from build123d import *

# Parameters (mm, degrees)
SKETCH1_R               = 50.8
SKETCH1_R_2             = 3.175
BOSS_EXTRUDE1_DEPTH     = 71.12
CUT_EXTRUDE1_DEPTH      = 102.09072361
CUT_EXTRUDE1_DEPTH_BACK = 102.09072361
SKETCH2_R               = 1.27
SKETCH7_R               = 2.5
CUT_EXTRUDE4_DEPTH      = 12.7
SKETCH8_R               = 15.748
SKETCH8_R_2             = 3.175
BOSS_EXTRUDE2_DEPTH     = 6.35
CUT_EXTRUDE6_DEPTH      = 4
SKETCH6_R               = 2.5
CUT_EXTRUDE7_DEPTH      = 7


with BuildPart() as part:
    # Sketch1 → Boss-Extrude1 (new body)
    with BuildSketch(Plane.XY):
        Circle(SKETCH1_R)
        Circle(SKETCH1_R_2, mode=Mode.SUBTRACT)
    extrude(amount=BOSS_EXTRUDE1_DEPTH)

    # Sketch2 → Cut-Extrude1 (cut, two sides: drawn at the far end of the back side and taken through both)
    with BuildSketch(Plane(origin=(0, 0, 0), x_dir=(0, 0, -1), z_dir=(1, 0, 0)).offset(-CUT_EXTRUDE1_DEPTH_BACK)):
        with Locations((-35.56, 38.1)):
            Circle(SKETCH2_R)
    extrude(amount=CUT_EXTRUDE1_DEPTH + CUT_EXTRUDE1_DEPTH_BACK, mode=Mode.SUBTRACT)

    # Sketch7 → Cut-Extrude4 (cut)
    with BuildSketch(Plane(origin=(0, 0, 0), x_dir=(-1, 0, 0), z_dir=(0, 0, -1))):
        with Locations((28.575, 0)):
            Circle(SKETCH7_R)
        with Locations((0, 28.575)):
            Circle(SKETCH7_R)
        with Locations((-28.575, 0)):
            Circle(SKETCH7_R)
        with Locations((0, -28.575)):
            Circle(SKETCH7_R)
    cut_extrude4 = extrude(amount=-CUT_EXTRUDE4_DEPTH, mode=Mode.SUBTRACT)

    # Mirror1: Cut-Extrude4 across plane
    add(cut_extrude4.mirror(Plane.XY.offset(35.56)), mode=Mode.SUBTRACT)

    # Sketch8 → Boss-Extrude2 (add)
    with BuildSketch(Plane.XY.offset(71.12)):
        Circle(SKETCH8_R)
        Circle(SKETCH8_R_2, mode=Mode.SUBTRACT)
    extrude(amount=BOSS_EXTRUDE2_DEPTH)

    # Sketch5 → Cut-Extrude6 (cut)
    with BuildSketch(Plane.XY.offset(77.47)):
        with BuildLine():
            Line((-4.330127019, 5.5), (4.330127019, 5.5))
            ThreePointArc((4.330127019, 5.5), (7, 0), (4.330127019, -5.5))
            Line((4.330127019, -5.5), (-4.330127019, -5.5))
            ThreePointArc((-4.330127019, -5.5), (-7, 0), (-4.330127019, 5.5))
        make_face()
    extrude(amount=-CUT_EXTRUDE6_DEPTH, mode=Mode.SUBTRACT)

    # Sketch6 → Cut-Extrude7 (cut)
    with BuildSketch(Plane.XY.offset(77.47)):
        with Locations((-8, 8)):
            Circle(SKETCH6_R)
        with Locations((8, 8)):
            Circle(SKETCH6_R)
        with Locations((8, -8)):
            Circle(SKETCH6_R)
        with Locations((-8, -8)):
            Circle(SKETCH6_R)
    extrude(amount=-CUT_EXTRUDE7_DEPTH, mode=Mode.SUBTRACT)

    # Sketch9 → Cut-Revolve1 (revolve, cut)
    with BuildSketch(Plane(origin=(0, 0, 0), x_dir=(0, 0, -1), z_dir=(1, 0, 0)), mode=Mode.PRIVATE) as cut_revolve1_sk:
        with BuildLine():
            Line((-71.12, 50.8), (-46.204077708, 45.460873794))
            ThreePointArc((-46.204077708, 45.460873794), (-35.56, 44.33323643), (-24.915922292, 45.460873794))
            Line((-24.915922292, 45.460873794), (0, 50.8))
            Line((0, 50.8), (-71.12, 50.8))
        make_face()
    revolve(cut_revolve1_sk.sketch.rotate(Axis((0, 0, -3.8735), (0, 0, 1)), 90), axis=Axis((0, 0, -3.8735), (0, 0, 1)), mode=Mode.SUBTRACT)


solid = part.part
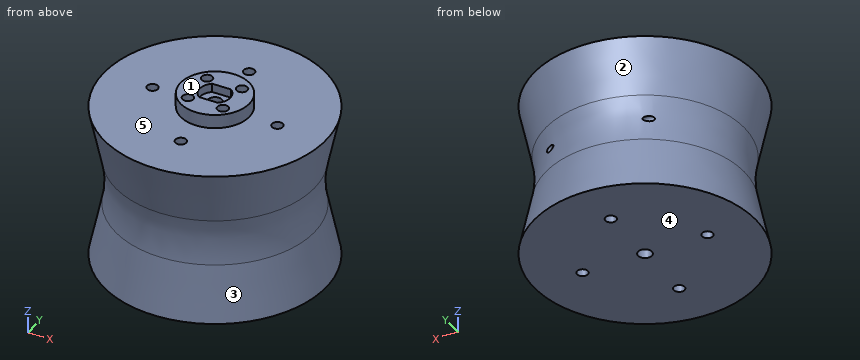
Could you check a few things on this model? Use its own coordinates, in mm. Face numbers are marked on the shaded views. A direction names the side the tool comes from. Round coordinates to 2 decimals unless told otherwise and drop trailing zeros. Write each loop counter-clockwise with the first axis right and the second up, starting at its lowest first coordinate (ties: lowest second). Pieces come first, ordered by that corner, then holes. Notation, with made-up numbers: (59.5, 6) - (117.5, 6) arc R25 ccw to (117.5, 29) - close; hole circle Ø4 at (13.5, 38.25). An arc over 180 degrees is marked (long way). Use a Markdown table: item, result.
Q1. Please list where these lines run through material, in increasing order: L1, parallel to Y at x = -8, z = 74.5; L2, parallel to Y at x = 9, z = 70.5; L3, parallel to Y at x = 0, z = 66.5 (3 decimals).
Output values:
| item | result |
|---|---|
| L1 | -13.56 to -10.5, -5.5 to 5.5, 10.5 to 13.56 |
| L2 | -49.86 to -10.29, -5.71 to 5.71, 10.29 to 49.86 |
| L3 | -49.81 to -31.075, -26.075 to -3.175, 3.175 to 26.075, 31.075 to 49.81 |
Q2. Thinking about a two-plate mould opening in Z: for the marked faces 3, 4 and 5, which applies, released by +Z, released by -Z, zero draft, split by the parting line, or undercut?
Output values:
| item | result |
|---|---|
| face 3 | undercut |
| face 4 | released by -Z |
| face 5 | released by +Z |
Q3. For pin 1 (4 mm diameter, centred on x = 0, y = 28.575, fed in from -Z); pin 2 (5.5 mm diameter, centred on x = -1, y = 28.5, fed in from +Z); pin 3 (1.5 mm diameter, centred on x = 28, z = 66.5, fed in from +Y), each with a flat end and sliding along its axis, tell me the tip position at first contact or that it passes through.
Output values:
| item | result |
|---|---|
| pin 1 | z = 12.7 |
| pin 2 | z = 71.12 |
| pin 3 | y = 41.73 |
Q4. I want a section at B-B (z = 56). List the corners of the cut face in (x, y) for me (3 decimals).
Output values:
| item | result |
|---|---|
| outline | circle Ø95.12 at (0, 0); hole circle Ø6.35 at (0, 0) |
Q5. I want a section at C-C (z = 19). List the corners of the cut face in (x, y) for me (3 decimals), plus the area to 3 significant figures.
Output values:
| item | result |
|---|---|
| outline | circle Ø93.457 at (0, 0); hole circle Ø6.35 at (0, 0) |
| area | 6,830 mm2 |
Q6. I want a section at A-A (z = 8). List the corners of the cut face in (x, y) for me (3 decimals).
Output values:
| item | result |
|---|---|
| outline | circle Ø98.171 at (0, 0); hole circle Ø5 at (-28.575, 0); hole circle Ø6.35 at (0, 0); hole circle Ø5 at (0, -28.575); hole circle Ø5 at (0, 28.575); hole circle Ø5 at (28.575, 0) |
Q7. For the marked faces 1 and 2, which set-ups out of +Z, -Z, +X, -X, +Y, -Y let a thin tool reach every point of the face, with its end or its side?
Output values:
| item | result |
|---|---|
| face 1 | +Z, +X, -X, +Y, -Y |
| face 2 | none |
